```python
from build123d import *

# Parameters (mm, degrees)
F1_DEPTH = 44
F2_R     = 2
F4_DEPTH = 10


with BuildPart() as f1:
    # F0 (on Front) → F1 (new body)
    with BuildSketch(Plane.XZ):
        with BuildLine():
            ThreePointArc((-68.716378, -9.5), (-61.998863, -6.717514), (-59.216378, 0))
            ThreePointArc((-59.216378, 0), (-61.998863, 6.717514), (-68.716378, 9.5))
            ThreePointArc((-68.716378, 9.5), (-78.216378, 0), (-68.716378, -9.5))
        make_face()
        with BuildLine():
            ThreePointArc((-68.716378, 9.5), (-61.998863, 6.717514), (-59.216378, 0))
            ThreePointArc((-59.216378, 0), (-61.998863, -6.717514), (-68.716378, -9.5))
            Line((-68.716378, -9.5), (56.283622, -9.5))
            Line((56.283622, -9.5), (56.283622, 9.5))
            Line((56.283622, 9.5), (-68.716378, 9.5))
        make_face()
    extrude(amount=F1_DEPTH)

    # F2
    f2_edges = [f1.edges().sort_by_distance(p)[0] for p in [
        (-6.216378, -44, 9.5),
        (56.283622, -22, 9.5),
        (56.283622, -22, -9.5),
        (56.283622, -44, 0),
        (56.283622, 0, 0),
        (-6.216378, 0, -9.5),
        (-6.216378, 0, 9.5),
    ]]
    fillet(f2_edges, radius=F2_R)

    # F3 (on face) → F4 (join)
    with BuildSketch(Plane(origin=(0, 0, 0), x_dir=(-1, 0, 0), z_dir=(0, 1, 0))):
        with BuildLine():
            ThreePointArc((68.716378, -7.5), (76.216378, 0), (68.716378, 7.5))
            Line((68.716378, 7.5), (68.716378, -7.5))
        make_face()
    extrude(amount=F4_DEPTH)


solid = f1.part
```
Model file for the job. Use its own axes, mm. A direction names the side the tool comes from. Give positions to 0.01 mm unless a question says otherwise; leave off trailing zeros. Write each loop counter-clockwise with the first axis right and the second up, starting at its lowest first coordinate (ties: lowest second). Pieces come first, ordered by that corner, then holes. Notation, with made-up numbers: (46, -25.75) - (97, -25.75) arc R28 cw to (97, -7.75) - close; hole circle Ø11 at (-22.5, 84.25). An arc over 180 degrees is marked (long way). One line per question, with ' | ' between items. Start each with the question number.
(1) 3-axis set-ups, long thin cutter, end or side, ignore diameter. For faces 1 (the face through (-6, -22, 9.5)), 2 (the face through (-8, 0, 0)), 3 (the face through (-76.215, 4.93, -0.165)): which of +Z, -Z, +X, -X, +Y, -Y reach the whole face in a straight line?
(2) Wall check: line 1 along Y through (x, z) = (-50, -5.75); line 2 along X through (y, z) = (-39.5, 4.5); line 3 along X through (y, z) = (-15, 5.75). Give the ranges that are in metal, low to high. Write a range as from..to.
(3) Slice it at B-B on z = 0. Write the cut outline in (x, y).
(4) Slice it at D-D on y = 4. Write the cut outline in (x, z).
(5) Slice it at C-C on y = -21.5. Write the cut outline in (x, z).
(6) Slice it at A-A on x = -9. Write the cut outline in (y, z), plus the area to 3 significant figures.
(7) Pin check, flat tips, straight feed: P1, Ø1.5, axis at y = -35, z = -3, coming from the -X side; P2, Ø10, axis at x = 38, y = 4.5, coming from the +Z side; P3, Ø7.5, axis at x = -1, z = 3, coming from the +Y side. Stop position of each tip, or through.
Results below:
1) face 1: +Z, +X, -X, +Y, -Y | face 2: +Z, -Z, +X, +Y | face 3: -X, +Y
2) line 1: -44..0 | line 2: -77.08..56.28 | line 3: -76.28..56.28
3) outline: (-78.22, -42) arc R2 ccw to (-76.22, -44) - (54.28, -44) arc R2 ccw to (56.28, -42) - (56.28, -2) arc R2 ccw to (54.28, 0) - (-68.72, 0) - (-68.72, 10) - (-76.22, 10) - (-76.22, 0) arc R2 ccw to (-78.22, -2) - close
4) outline: (-68.72, -7.5) - (-68.72, 7.5) arc R7.5 ccw to start
5) outline: (-68.72, -9.5) - (54.28, -9.5) arc R2 ccw to (56.28, -7.5) - (56.28, 7.5) arc R2 ccw to (54.28, 9.5) - (-68.72, 9.5) arc R9.5 ccw to start
6) outline: (-44, -7.5) arc R2 ccw to (-42, -9.5) - (-2, -9.5) arc R2 ccw to (0, -7.5) - (0, 7.5) arc R2 ccw to (-2, 9.5) - (-42, 9.5) arc R2 ccw to (-44, 7.5) - close | area: 833 mm^2
7) P1: x = -77.95 | P2: z = 8.82 | P3: y = 0
